Work out the finished part from the listing and answer in its coordinate system (mm). A direction names the side the tool comes from. Round coordinates to 2 decimals unless told otherwise and drop trailing zeros. Order: outer loops, then holes, each group sorted by start corner. A loop starts at its lowest first (then second) coordinate and runs counter-clockwise, first axis right, second up. Notation, with made-up numbers: (75, 81) - (102, 81) arc R23 cw to (102, 99) - close; hole circle Ø7 at (10.25, 64). An arc over 180 degrees is marked (long way). Use CSV: the item, a comma, the result in double quotes.
from build123d import *

# Parameters (mm, degrees)
SKETCH1_W           = 21.8
SKETCH1_H           = 22.6
BOSS_EXTRUDE1_DEPTH = 11.4
SKETCH2_W           = 31.8
SKETCH2_H           = 1.555593414
BOSS_EXTRUDE2_DEPTH = 11.4
SKETCH3_R           = 5.7
BOSS_EXTRUDE3_DEPTH = 3
SKETCH4_R           = 2.275
BOSS_EXTRUDE4_DEPTH = 2
SKETCH5_R           = 0.717779634
CUT_EXTRUDE1_DEPTH  = 2.4
SKETCH7_R           = 1.5
CUT_EXTRUDE2_DEPTH  = 10


with BuildPart() as part:
    # Sketch1 → Boss-Extrude1 (new body)
    with BuildSketch(Plane.XY):
        Rectangle(SKETCH1_W, SKETCH1_H)
    extrude(amount=BOSS_EXTRUDE1_DEPTH)

    # Sketch2 → Boss-Extrude2 (add)
    with BuildSketch(Plane.XY.offset(11.4)):
        with Locations((0, 9.475117961)):
            Rectangle(SKETCH2_W, SKETCH2_H)
    extrude(amount=-BOSS_EXTRUDE2_DEPTH)

    # Sketch3 → Boss-Extrude3 (add)
    with BuildSketch(Plane(origin=(0, 11.3, 0), x_dir=(1, 0, 0), z_dir=(0, 1, 0))):
        with Locations(Location((5.2, -5.7, 0), (0, 0, 270))):
            Circle(SKETCH3_R)
    extrude(amount=BOSS_EXTRUDE3_DEPTH)

    # Sketch4 → Boss-Extrude4 (add)
    with BuildSketch(Plane(origin=(0, 14.3, 0), x_dir=(1, 0, 0), z_dir=(0, 1, 0))):
        with Locations(Location((5.2, -5.7, 0), (0, 0, 270))):
            Circle(SKETCH4_R)
    extrude(amount=BOSS_EXTRUDE4_DEPTH)

    # Sketch5 → Cut-Extrude1 (cut)
    with BuildSketch(Plane(origin=(0, 16.3, 0), x_dir=(1, 0, 0), z_dir=(0, 1, 0))):
        with Locations(Location((5.2, -5.7, 0), (0, 0, 270))):
            Circle(SKETCH5_R)
    extrude(amount=-CUT_EXTRUDE1_DEPTH, mode=Mode.SUBTRACT)

    # Sketch7 → Cut-Extrude2 (cut)
    with BuildSketch(Plane(origin=(0, 10.252914668, 0), x_dir=(1, 0, 0), z_dir=(0, 1, 0))):
        with Locations(Location((13.399999972, -5.699036205, 0), (0, 0, 270))):
            Circle(SKETCH7_R)
        with Locations(Location((-13.4, -5.7, 0), (0, 0, 270))):
            Circle(SKETCH7_R)
    extrude(amount=-CUT_EXTRUDE2_DEPTH, mode=Mode.SUBTRACT)


solid = part.part
(1) Find section A-A (x = 13.4). Determine the outline of the cut face in (y, z), and give its area (3 significant figures).
Findings below:
outline,"(8.7, 0) - (10.25, 0) - (10.25, 4.2) - (8.7, 4.2) - close; (8.7, 7.2) - (10.25, 7.2) - (10.25, 11.4) - (8.7, 11.4) - close"
area,"13.1 mm²"
(2) Each of these flat-tipped pins is pushed along its axis until it touches: pin 1 (4 mm diameter, centred on x = -14, z = 4.5, fed in from +Y); pin 2 (4 mm diameter, centred on y = 5.5, z = 2, fed in from +X); pin 3 (1.7 mm diameter, centred on x = 7, z = 8.5, fed in from +Y); pin 4 (2.5 mm diameter, centred on x = -13.4, z = 5.7, fed in from -Y). Where does it stop, or does it pass through?
Findings below:
pin 1,"stops at y = 10.25"
pin 2,"stops at x = 10.9"
pin 3,"stops at y = 14.3"
pin 4,"passes through"
(3) Find the intervals of material crossed by L1, parallel to X at y = 9.5, z = 5.7; L2, parallel to X at y = 14.55, z = 5.7 (3 decimals); L3, parallel to Y at x = 10.5, z = 8.25, in increasing order. Write a range as from..to.
Findings below:
L1,"x = -15.9..-14.9, -11.9..11.9, 14.9..15.9"
L2,"x = 2.925..4.482, 5.918..7.475"
L3,"y = -11.3..11.3"
(4) Find section C-C (x = 4). Determine the outline of the cut face in (y, z).
Findings below:
outline,"(-11.3, 0) - (11.3, 0) - (11.3, 0.13) - (14.3, 0.13) - (14.3, 3.77) - (16.3, 3.77) - (16.3, 7.63) - (14.3, 7.63) - (14.3, 11.27) - (11.3, 11.27) - (11.3, 11.4) - (-11.3, 11.4) - close"
(5) The mould has two halves that part along X. Classify faces 1 (the flat face through (-10.9, 11, 6)), 2 (the cylindrical face through (12.07, 9.49, 6.39)), 3 (the cylindrical face through (10.01, 12.78, 8.76)): released by +X, released by -X, zero draft, split by the parting line, or undercut.
Findings below:
face 1,"released by -X"
face 2,"undercut"
face 3,"split by the parting line"
(6) Find section B-B (y = -9). Determine the outline of the cut face in (x, z).
Findings below:
outline,"(-10.9, 0) - (10.9, 0) - (10.9, 11.4) - (-10.9, 11.4) - close"
(7) Find section D-D (x = 8). Determine the outline of the cut face in (y, z), and give its area (3 significant figures).
Findings below:
outline,"(-11.3, 0) - (11.3, 0) - (11.3, 0.74) - (14.3, 0.74) - (14.3, 10.66) - (11.3, 10.66) - (11.3, 11.4) - (-11.3, 11.4) - close"
area,"287 mm²"
(8) For faces 4 (the cylindrical face through (5.232, 15.117, 4.983)), 5 (the flat face through (-15.1, 10.253, 5.8)), 6 (the flat face through (10, 11.3, 1)), 7 (the flat face through (-10.9, -1, 6)), 8 (the flat face through (10, 11.3, 10)), determine the directions among +Z, -Z, +X, -X, +Y, -Y from which every point of the face is accessible in a straight line to the end or side of a thin tool.
Findings below:
face 4,"+Y"
face 5,"+Z, -Z, -X, +Y"
face 6,"-Z, +X, +Y"
face 7,"+Z, -Z, -X, -Y"
face 8,"+Z, +X, +Y"
